Read the model definition and answer for the solid it produces. Units are mm, in the model's axes. A direction names the side the tool comes from. Give positions to 0.01 mm unless a question says otherwise; leave off trailing zeros. Order: outer loops, then holes, each group sorted by start corner. A loop starts at its lowest first (then second) coordinate and runs counter-clockwise, first axis right, second up. Notation, with made-up numbers: (3.25, 88) - (29.25, 88) arc R35 cw to (29.25, 122) - close; hole circle Ø3 at (85.5, -6.5). An arc over 180 degrees is marked (long way). Write each question's results on one line, items separated by ' | '.
from build123d import *

# Parameters (mm, degrees)
ESBO_O2_W                = 60.1
ESBO_O2_H                = 60
ESBO_O2_W_2              = 58.1
ESBO_O2_H_2              = 58
RESSALTO_EXTRUS_O3_DEPTH = 240
ESBO_O4_R                = 2
ESBO_O4_R_2              = 2.5
CORTE_EXTRUS_O1_DEPTH    = 246.345874994
CORTE_EXTRUS_O2_DEPTH    = 10


with BuildPart() as part:
    # Esboço2 → Ressalto-extrusão3 (new body)
    with BuildSketch(Plane(origin=(0, 0, 0), x_dir=(0, 0, -1), z_dir=(1, 0, 0))):
        with Locations((0.05, 11.092436975)):
            Rectangle(ESBO_O2_W, ESBO_O2_H)
        with Locations((0.05, 11.092436975)):
            Rectangle(ESBO_O2_W_2, ESBO_O2_H_2, mode=Mode.SUBTRACT)
    extrude(amount=RESSALTO_EXTRUS_O3_DEPTH)

    # Esboço4 → Corte-extrusão1 (cut, through all)
    with BuildSketch(Plane(origin=(0, 0, 0), x_dir=(1, 0, 0), z_dir=(0, 1, 0))):
        with Locations(Location((12, 15, 0), (0, 0, 270))):
            Circle(ESBO_O4_R)
        with Locations(Location((12, -15, 0), (0, 0, 270))):
            Circle(ESBO_O4_R)
        with Locations(Location((42, -15, 0), (0, 0, 270))):
            Circle(ESBO_O4_R)
        with Locations(Location((42, 15, 0), (0, 0, 270))):
            Circle(ESBO_O4_R)
        with Locations(Location((210, -21, 0), (0, 0, 270))):
            Circle(ESBO_O4_R_2)
        with Locations(Location((210, 21, 0), (0, 0, 270))):
            Circle(ESBO_O4_R_2)
        with Locations(Location((99, -21, 0), (0, 0, 270))):
            Circle(ESBO_O4_R_2)
        with Locations(Location((99, 21, 0), (0, 0, 270))):
            Circle(ESBO_O4_R_2)
    extrude(amount=-CORTE_EXTRUS_O1_DEPTH, mode=Mode.SUBTRACT)

    # Esboço5 → Corte-extrusão2 (cut)
    with BuildSketch(Plane.XY.offset(30)):
        with BuildLine():
            Line((194.051333541, 1.259947871), (114.051333541, 1.259947871))
            ThreePointArc((114.051333541, 1.259947871), (100.718844437, 14.592436975), (114.051333541, 27.924926079))
            Line((114.051333541, 27.924926079), (194.051333541, 27.924926079))
            ThreePointArc((194.051333541, 27.924926079), (207.383822645, 14.592436975), (194.051333541, 1.259947871))
        make_face()
    extrude(amount=-CORTE_EXTRUS_O2_DEPTH, mode=Mode.SUBTRACT)


solid = part.part
(1) Section B-B (x = 210) is taken. Give the vertices of the cut face in (y, z), plus the area to 3 significant figures.
Conclusion:
outline: (-18.91, -30.1) - (41.09, -30.1) - (41.09, 30) - (-18.91, 30) - (-18.91, 23.5) - (-17.91, 23.5) - (-17.91, 29) - (40.09, 29) - (40.09, -29.1) - (-17.91, -29.1) - (-17.91, -23.5) - (-18.91, -23.5) - close; (-18.91, -18.5) - (-17.91, -18.5) - (-17.91, 18.5) - (-18.91, 18.5) - close | area: 226 mm^2
(2) Section C-C (z = 21) is taken. Give the vertices of the cut face in (x, y), plus the area to 3 significant figures.
Conclusion:
outline: (0, -18.91) - (96.5, -18.91) - (96.5, -17.91) - (0, -17.91) - close; (0, 40.09) - (240, 40.09) - (240, 41.09) - (0, 41.09) - close; (101.5, -18.91) - (207.5, -18.91) - (207.5, -17.91) - (101.5, -17.91) - close; (212.5, -18.91) - (240, -18.91) - (240, -17.91) - (212.5, -17.91) - close | area: 470 mm^2
(3) Section D-D (y = 17) is taken. Give the vertices of the cut face in (x, z), plus the area to 3 significant figures.
Conclusion:
outline: (0, -30.1) - (240, -30.1) - (240, -29.1) - (0, -29.1) - close; (0, 29) - (100.94, 29) - (100.94, 30) - (0, 30) - close; (207.16, 29) - (240, 29) - (240, 30) - (207.16, 30) - close | area: 374 mm^2
(4) Section A-A (z = -10.5) is taken. Give the vertices of the cut face in (x, y), plus the area to 3 significant figures.
Conclusion:
outline: (0, -18.91) - (240, -18.91) - (240, -17.91) - (0, -17.91) - close; (0, 40.09) - (240, 40.09) - (240, 41.09) - (0, 41.09) - close | area: 480 mm^2
(5) For faces 5 (the face through (100.722, 14.299, 29.507)), 6 (the face through (212.48, -18.4, 20.67)), 7 (the face through (118, -17.908, 0)), determine the directions among +Z, -Z, +X, -X, +Y, -Y from which every point of the face is accessible in a straight line to the end or side of a thin tool.
Conclusion:
face 5: +Z | face 6: -Y | face 7: +X, -X
(6) Each of these flat-tipped pins is pushed along its axis until it touches: pin 1 (12 mm diameter, centred on y = 32.5, z = -0.5, fed in from +X); pin 2 (4 mm diameter, centred on x = 99, z = 21, fed in from -Y). Where does it stop, or does it pass through?
Conclusion:
pin 1: through | pin 2: y = 40.09
(7) The mould has two halves that part along Z. Classify faces 1 (the face through (118, -3, 30)), 2 (the face through (118, 11, -30.1)), 3 (the face through (118, 41.092, 0)), 4 (the face through (13.983, -18.401, -15.26)): pulls with the +Z half, pulls with the -Z half, needs draft (parallel to the pull), parting line crosses it, or undercut.
Conclusion:
face 1: pulls with the +Z half | face 2: pulls with the -Z half | face 3: needs draft | face 4: undercut
(8) Consider probe 1 along X at (y, z) = (-18.45, -21); probe 2 along X at (y, z) = (-18.15, -15); probe 3 along Y at (x, z) = (62, -3). Determine where each line is inside the solid, lowest interval first. Write a range as [from, to].
Conclusion:
probe 1: [0, 96.5], [101.5, 207.5], [212.5, 240] | probe 2: [0, 10], [14, 40], [44, 240] | probe 3: [-18.91, -17.91], [40.09, 41.09]
